CAD build for the part. Positions are in the model's coordinates, mm. A direction names the side the tool comes from. Give positions to 0.01 mm unless a question says otherwise; leave off trailing zeros. Loops run counter-clockwise (first coordinate to the right, second up) from the corner with the lowest first, then second, coordinate; pieces in that order, holes last. Notation, with made-up numbers: (-37.5, 31) - (15.5, 31) arc R13 ccw to (15.5, 51) - close; hole circle Ø7 at (43.5, -8). An arc over 180 degrees is marked (long way). Return JSON: item names as keys, results as strings.
from build123d import *

# Parameters (mm, degrees)
EXTRUDE_1_DEPTH     = 130
SKETCH_2_W          = 6
SKETCH_2_H          = 6
CUT_EXTRUDE_1_DEPTH = 15


with BuildPart() as part:
    # 草图1 → 凸台-拉伸1 (new body)
    with BuildSketch(Plane(origin=(0, 0, 0), x_dir=(0, 0, -1), z_dir=(1, 0, 0))):
        with BuildLine():
            Line((-1.5, 14.924811557), (-1.5, 0))
            Line((-1.5, 0), (1.5, 0))
            Line((1.5, 0), (1.5, 14.924811557))
            ThreePointArc((1.5, 14.924811557), (0, 15), (-1.5, 14.924811557))
        make_face()
        with BuildLine():
            Line((1.5, 0), (-1.5, 0))
            Line((-1.5, 0), (-1.5, 14.924811557))
            ThreePointArc((-1.5, 14.924811557), (-10.062305899, -11.124297731), (15, 0))
            ThreePointArc((15, 0), (11.124297731, 10.062305899), (1.5, 14.924811557))
            Line((1.5, 14.924811557), (1.5, 0))
        make_face()
        with BuildLine():
            Line((-1.5, 17), (-1.5, 14.924811557))
            ThreePointArc((-1.5, 14.924811557), (0, 15), (1.5, 14.924811557))
            Line((1.5, 14.924811557), (1.5, 17))
            Line((1.5, 17), (-1.5, 17))
        make_face()
    extrude(amount=EXTRUDE_1_DEPTH)

    # 草图2 → 切除-拉伸1 (cut)
    with BuildSketch(Plane(origin=(130, 0, 0), x_dir=(0, 0, -1), z_dir=(1, 0, 0))):
        Rectangle(SKETCH_2_W, SKETCH_2_H)
    extrude(amount=-CUT_EXTRUDE_1_DEPTH, mode=Mode.SUBTRACT)


solid = part.part
1. Cut at B-B, the plane x = 32.5. Write the cut outline in (y, z), plus the area to 3 significant figures.
Values follow:
{"outline": "(14.92, -1.5) - (17, -1.5) - (17, 1.5) - (14.92, 1.5) arc R15 ccw (long way) to start", "area": "713 mm²"}
2. Cut at C-C, the plane y = -1.5. Write the cut outline in (x, z).
Values follow:
{"outline": "(0, -14.92) - (130, -14.92) - (130, -3) - (115, -3) - (115, 3) - (130, 3) - (130, 14.92) - (0, 14.92) - close"}
3. Drill centre lines: probe 1 along Y at (x, z) = (26, -0.5); probe 2 along Z at (x, y) = (57.5, -0.5); probe 3 along Z at (x, y) = (114.5, -11). Where is each one in solid material? Low to high.
Values follow:
{"probe 1": "y = -14.99 to 17", "probe 2": "z = -14.99 to 14.99", "probe 3": "z = -10.2 to 10.2"}
4. Cut at A-A, the plane z = 0. Write the cut outline in (x, y), plus the area to 3 significant figures.
Values follow:
{"outline": "(0, -15) - (130, -15) - (130, -3) - (115, -3) - (115, 3) - (130, 3) - (130, 17) - (0, 17) - close", "area": "4,070 mm²"}
5. Which spindle directions (+Z, -Z, +X, -X, +Y, -Y) get a long thin tool onto all of the face, cutting with end or side? Do faces 1 (the face through (123, -3, 0)), 2 (the face through (0, 1, 0)). Say none if no direction does.
Values follow:
{"face 1": "+X", "face 2": "+Z, -Z, -X, +Y, -Y"}
6. Drop flat-ended pins along their axis: P1, Ø0.6, axis at x = 34.5, y = 15.5, coming from the -Z side; P2, Ø1.5, axis at x = 28, z = 6.5, coming from the +Y side; P3, Ø1.5, axis at x = 68.5, y = 2, coming from the -Z side. Give the stop position or say it passes through.
Values follow:
{"P1": "stops at z = -1.5", "P2": "stops at y = 13.85", "P3": "stops at z = -14.95"}
7. Pull direction Z, two halves, no side cores. Call faces 3 (the face through (64, 16, 1.5)), 4 (the face through (64, 16, -1.5)), 5 (the face through (123, 3, 0)), 6 (the face through (130, 1, 4)): +Z half, -Z half, draft (parallel to the pull), parting line (faces both ways), or undercut.
Values follow:
{"face 3": "+Z half", "face 4": "-Z half", "face 5": "undercut", "face 6": "draft"}
8. Cut at D-D, the plane z = -9. Write the cut outline in (x, y), plus the area to 3 significant figures.
Values follow:
{"outline": "(0, -12) - (130, -12) - (130, 12) - (0, 12) - close", "area": "3,120 mm²"}
